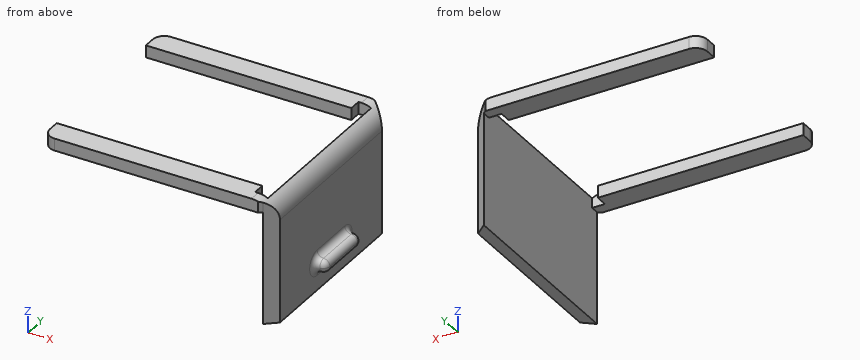
```python
from build123d import *

# Parameters (mm, degrees)
BOSS_EXTRUDE1_DEPTH = 29.3184
BOSS_EXTRUDE2_DEPTH = 2.8448
FILLET1_R           = 5
SKETCH3_W           = 3
SKETCH3_H           = 14
BOSS_EXTRUDE3_DEPTH = 3
FILLET2_R           = 1.5
FILLET3_R           = 1.5


# Some blends are built 0.0001 mm under size
with BuildPart() as part:
    # Sketch1 → Boss-Extrude1 (new body)
    with BuildSketch(Plane.XY):
        Polygon((33.95, 21.346198616), (33.95, -23.846198616), (36.648979486, -21.581485925), (36.648979486, -1.25), (36.648979486, 19.081485925), align=None)
    extrude(amount=BOSS_EXTRUDE1_DEPTH)

    # Sketch2 → Boss-Extrude2 (add)
    with BuildSketch(Plane.XY.offset(29.3184)):
        with BuildLine():
            Line((33.95, -21.846198616), (33.95, -23.846198616))
            Line((33.95, -23.846198616), (33.200504516, -24.4751))
            Line((33.200504516, -24.4751), (-14.764, -24.4751))
            ThreePointArc((-14.764, -24.4751), (-16.701369719, -23.67255493), (-17.503709057, -21.7351))
            Line((-17.503709057, -21.7351), (-17.503709057, -19.0141))
            Line((-17.503709057, -19.0141), (30.95, -19.0141))
            Line((30.95, -19.0141), (30.95, -21.846198616))
            Line((30.95, -21.846198616), (33.95, -21.846198616))
        make_face()
        with BuildLine():
            Line((30.95, 19.346198616), (33.95, 19.346198616))
            Line((33.95, 19.346198616), (33.95, 21.346198616))
            Line((33.95, 21.346198616), (33.200504516, 21.9751))
            Line((33.200504516, 21.9751), (-14.764, 21.9751))
            ThreePointArc((-14.764, 21.9751), (-16.701369719, 21.17255493), (-17.503709057, 19.2351))
            Line((-17.503709057, 19.2351), (-17.503709057, 16.5141))
            Line((-17.503709057, 16.5141), (30.95, 16.5141))
            Line((30.95, 16.5141), (30.95, 19.346198616))
        make_face()
    extrude(amount=-BOSS_EXTRUDE2_DEPTH)

    # Fillet1
    # the kernel refuses this fillet: 5 mm, written as the material it takes off along each edge
    with BuildSketch(Plane(origin=(36.648979486, 31.581485925, 29.3184), x_dir=(0, 0, -1), z_dir=(0, -1, 0))) as fillet1_piece_1:
        with BuildLine():
            CenterArc((FILLET1_R, -FILLET1_R), FILLET1_R, 90, 90)
            Line((0, -FILLET1_R), (0, 0))
            Line((0, 0), (FILLET1_R, 0))
        make_face()
    extrude(amount=65.66297185, mode=Mode.SUBTRACT)

    # Sketch3 → Boss-Extrude3 (add)
    with BuildSketch(Plane(origin=(36.648979486, 0, 0), x_dir=(0, 0, -1), z_dir=(1, 0, 0))):
        with Locations((-6.5, -1.25)):
            Rectangle(SKETCH3_W, SKETCH3_H)
    extrude(amount=BOSS_EXTRUDE3_DEPTH)

    # Fillet2
    fillet2_edges = [part.edges().sort_by_distance(p)[0] for p in [
        (39.648979486, -1.25, 8),
        (39.648979486, -8.25, 6.5),
        (39.648979486, -1.25, 5),
        (39.648979486, 5.75, 6.5),
    ]]
    fillet(fillet2_edges, radius=FILLET2_R - 0.0001)  # a hair under: the kernel refuses the full size

    # Fillet3
    # the kernel refuses this fillet: 1.5 mm, written as the material it takes off along each edge
    with BuildSketch(Plane(origin=(39.648979486, -6.75, 6.5), x_dir=(0, -1, 0), z_dir=(0, 0, 1))) as fillet3_piece_1:
        with BuildLine():
            CenterArc((0.0001, -1.4999), 1.4999, 0, 90)
            Line((1.5, -1.4999), (1.5, 0))
            Line((1.5, 0), (0.0001, 0))
        make_face()
    revolve(axis=Axis((39.648979486, -6.75, 6.5), (1, 0, 0)), revolution_arc=90, mode=Mode.SUBTRACT)
    with BuildSketch(Plane(origin=(39.648979486, -6.75, 6.5), x_dir=(0, 0, 1), z_dir=(0, 1, 0))) as fillet3_piece_2:
        with BuildLine():
            CenterArc((0.0001, -1.4999), 1.4999, 0, 90)
            Line((1.5, -1.4999), (1.5, 0))
            Line((1.5, 0), (0.0001, 0))
        make_face()
    revolve(axis=Axis((39.648979486, -6.75, 6.5), (1, 0, 0)), revolution_arc=90, mode=Mode.SUBTRACT)
    with BuildSketch(Plane(origin=(39.648979486, 4.25, 6.5), x_dir=(0, 0, -1), z_dir=(0, -1, 0))) as fillet3_piece_3:
        with BuildLine():
            CenterArc((0.0001, -1.4999), 1.4999, 0, 90)
            Line((1.5, -1.4999), (1.5, 0))
            Line((1.5, 0), (0.0001, 0))
        make_face()
    revolve(axis=Axis((39.648979486, 4.25, 6.5), (1, 0, 0)), revolution_arc=90, mode=Mode.SUBTRACT)
    with BuildSketch(Plane(origin=(39.648979486, 4.25, 6.5), x_dir=(0, 1, 0), z_dir=(0, 0, -1))) as fillet3_piece_4:
        with BuildLine():
            CenterArc((0.0001, -1.4999), 1.4999, 0, 90)
            Line((1.5, -1.4999), (1.5, 0))
            Line((1.5, 0), (0.0001, 0))
        make_face()
    revolve(axis=Axis((39.648979486, 4.25, 6.5), (1, 0, 0)), revolution_arc=90, mode=Mode.SUBTRACT)
    with BuildSketch(Plane(origin=(36.648979486, 5.75, 8), x_dir=(0, -1, 0), z_dir=(1, 0, 0)), Plane(origin=(36.648979486, 5.75, 5), x_dir=(0, 0, 1), z_dir=(1, 0, 0))) as fillet3_piece_5:
        with BuildLine():
            CenterArc((FILLET3_R, FILLET3_R), FILLET3_R, 180, 90)
            Line((0, FILLET3_R), (-FILLET3_R * 0.02, FILLET3_R))
            Line((-FILLET3_R * 0.02, FILLET3_R), (-FILLET3_R * 0.02, -FILLET3_R * 0.02))
            Line((-FILLET3_R * 0.02, -FILLET3_R * 0.02), (FILLET3_R, -FILLET3_R * 0.02))
            Line((FILLET3_R, -FILLET3_R * 0.02), (FILLET3_R, 0))
        make_face()
    extrude(amount=3, mode=Mode.SUBTRACT)
    with BuildSketch(Plane(origin=(36.648979486, -8.25, 5), x_dir=(0, 0, 1), z_dir=(1, 0, 0)), Plane(origin=(36.648979486, -8.25, 8), x_dir=(0, 1, 0), z_dir=(1, 0, 0))) as fillet3_piece_6:
        with BuildLine():
            CenterArc((FILLET3_R, -FILLET3_R), FILLET3_R, 90, 90)
            Line((0, -FILLET3_R), (-FILLET3_R * 0.02, -FILLET3_R))
            Line((-FILLET3_R * 0.02, -FILLET3_R), (-FILLET3_R * 0.02, FILLET3_R * 0.02))
            Line((-FILLET3_R * 0.02, FILLET3_R * 0.02), (FILLET3_R, FILLET3_R * 0.02))
            Line((FILLET3_R, FILLET3_R * 0.02), (FILLET3_R, 0))
        make_face()
    extrude(amount=3, mode=Mode.SUBTRACT)
    fillet3_2_edges = [part.edges().sort_by_distance(p)[0] for p in [
        (36.648979486, -1.25, 8),
        (36.648979486, -1.25, 5),
    ]]
    fillet(fillet3_2_edges, radius=FILLET3_R)


solid = part.part
```
Can you work these out from the model? Positions are in its coordinate system, mm. Coordinates: 2 decimals unless noted, no trailing zeros. Write each loop counter-clockwise with the first axis right and the second up, starting at its lowest first coordinate (ties: lowest second). Pieces come first, ordered by that corner, then holes. Notation, with made-up numbers: (-36, 11.25) - (-28, 11.25) arc R12 cw to (-28, 32.25) - close; hole circle Ø6 at (21, -24.5). An arc over 180 degrees is marked (long way). Return JSON: item names as keys, results as strings.
Q1. Please list where these lines run through material, in increasing order: L1, parallel to X at y = -8.5, z = 20; L2, parallel to Z at x = 21, y = 19.5; L3, parallel to X at y = -22, z = 5.5. Write a range as from..to.
Computed values:
{"L1": "x = 33.95..36.65", "L2": "z = 26.47..29.32", "L3": "x = 33.95..36.15"}
Q2. I'm going to push flat-ended pins straight in: pin 1 Ø2 at (y, z) = (16, 16) entering from +X; pin 2 Ø3 at (y, z) = (-20, 28.5) entering from +X; pin 3 Ø4.5 at (x, y) = (4, -22.5) entering from -Z. Where does each tip first touch, or does it pass through?
Computed values:
{"pin 1": "stops at x = 36.65", "pin 2": "stops at x = 35.87", "pin 3": "stops at z = 26.47"}
Q3. If we section it at D-D (y = 13.5): Please give me the cut outline in (x, z), then the cut area to 3 significant figures.
Computed values:
{"outline": "(33.95, 0) - (36.65, 0) - (36.65, 24.32) arc R5 ccw to (33.95, 28.76) - close", "area": "74.2 mm2"}
Q4. If we section it at C-C (z = 12.25): Please give me the cut outline in (x, y), then the cut area to 3 significant figures.
Computed values:
{"outline": "(33.95, -23.85) - (36.65, -21.58) - (36.65, 19.08) - (33.95, 21.35) - close", "area": "116 mm2"}
Q5. If we section it at A-A (x = 4): Please give me the cut outline in (y, z).
Computed values:
{"outline": "(-24.48, 26.47) - (-19.01, 26.47) - (-19.01, 29.32) - (-24.48, 29.32) - close; (16.51, 26.47) - (21.98, 26.47) - (21.98, 29.32) - (16.51, 29.32) - close"}
